Could you check a few things on this drawing? It's one solid part, dimensions in mm from its lowest x, y, z. Give positions to 0.01 mm unless a question says otherwise; leave off trailing zeros. Loops run counter-clockwise (first coordinate to the right, second up) from the corner with the lowest first, then second, coordinate; pieces in that order, holes last.
Q1. I need wall thicknesses on probe 1 along Z at (x, y) = (6.35, 2.85); probe 2 along Z at (x, y) = (5.5, 3.95); probe 3 along X at (y, z) = (4.55, 10.75). Which ranges of each line are inside material? Lowest first, please.
Q2. Suppose I cut it at C-C (y = 4.5). List the corners of the cut face in (x, z) for me, and give its area (3 significant figures).
Q3. Thinking about a two-plate mould opening in Z: for the marked faces 1, 2 and 3, which applies, pulls with the +Z half, pulls with the -Z half, needs draft (parallel to the pull), parting line crosses it, or undercut?
Q4. Suppose I cut it at B-B (x = 6.35). List the corners of the cut face in (y, z) for me.
Q5. Suppose I cut it at A-A (z = 13.97). List the corners of the cut face in (x, y) for me.
Q6. I'm going to push a flat-ended pin straight in: P1, Ø1, axis at x = 11.5, y = 2.5, coming from the +Z side. Where does the tip first touch, or does it pass through?
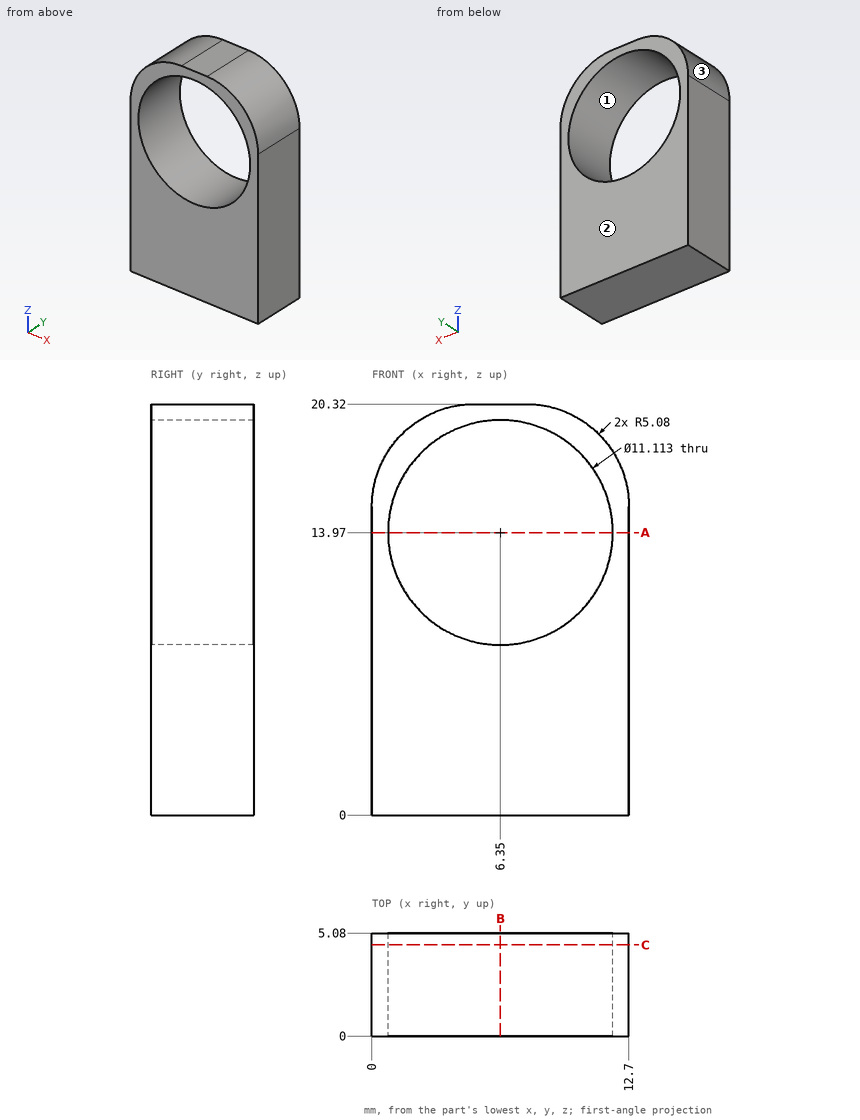
Solutions:
1. probe 1: z = 0 to 8.41, 19.53 to 20.32
1. probe 2: z = 0 to 8.48, 19.46 to 20.32
1. probe 3: x = 0 to 1.82, 10.88 to 12.7
2. outline: (0, 0) - (12.7, 0) - (12.7, 15.24) arc R5.08 ccw to (7.62, 20.32) - (5.08, 20.32) arc R5.08 ccw to (0, 15.24) - close; hole circle Ø11.11 at (6.35, 13.97)
2. area: 150 mm2
3. face 1: undercut
3. face 2: needs draft
3. face 3: pulls with the +Z half
4. outline: (0, 0) - (5.08, 0) - (5.08, 8.41) - (0, 8.41) - close; (0, 19.53) - (5.08, 19.53) - (5.08, 20.32) - (0, 20.32) - close
5. outline: (0, 0) - (0.79, 0) - (0.79, 5.08) - (0, 5.08) - close; (11.91, 0) - (12.7, 0) - (12.7, 5.08) - (11.91, 5.08) - close
6. P1: stops at z = 19.03
